from build123d import *

# Parameters (mm, degrees)
F1_DEPTH = 406.4
F2_R     = 1.27
F4_D     = 4.318
F4_DEPTH = 25.4
F4_TIP   = 1.2972580765


with BuildPart() as f1:
    # F0 (on Top) → F1 (new body)
    with BuildSketch(Plane.XY):
        Polygon((12.7, 0), (0, 0), (-12.7, 0), (-12.7, -3.175), (-1.5875, -3.175), (-1.5875, -12.7), (0, -12.7), (1.5875, -12.7), (1.5875, -3.175), (12.7, -3.175), align=None)
    extrude(amount=F1_DEPTH)

    # F2
    f2_edges = [f1.edges().sort_by_distance(p)[0] for p in [
        (-1.5875, -3.175, 203.2),
        (1.5875, -3.175, 203.2),
    ]]
    fillet(f2_edges, radius=F2_R)

    # F4
    with Locations(Plane(origin=(0, 0, 0), x_dir=(-1, 0, 0), z_dir=(0, 1, 0))):
        with Locations((-6.35, 400.05), (-6.35, 387.35), (6.35, 387.35), (6.35, 400.05), (-6.35, 6.35), (-6.35, 19.05), (6.35, 19.05), (6.35, 6.35)):
            Hole(F4_D / 2, depth=F4_DEPTH)
            with Locations((0, 0, -(F4_DEPTH + F4_TIP / 2))):  # 118° drill point
                Cone(0, F4_D / 2, F4_TIP, mode=Mode.SUBTRACT)


solid = f1.part
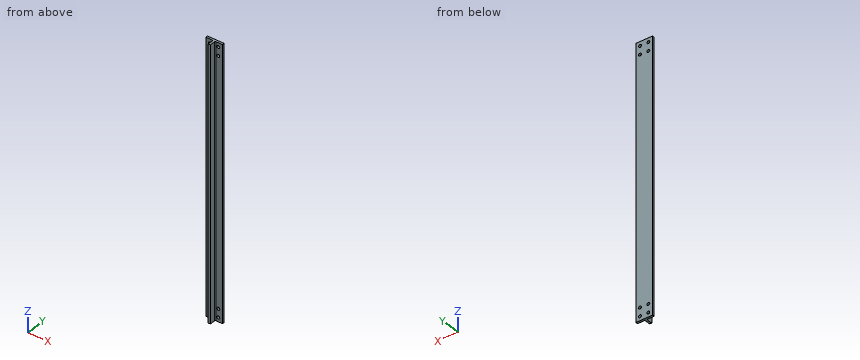
Source: CAD feature listing. Evaluate the final solid. Frame: model axes, mm. Coordinates: 2 decimals unless noted, no trailing zeros. Loops run counter-clockwise (first coordinate to the right, second up) from the corner with the lowest first, then second, coordinate; pieces in that order, holes last. Notation, with made-up numbers: (2, 19) -> (23, 19) arc R27 cw to (23, 45) -> close; hole circle Ø3 at (-14, 36). An arc over 180 degrees is marked (long way). Answer in a Markdown table with one row per item. Add a question column.
Q1. Contact query for flat-ended pins moving along their axis: pin 1 Ø5 at (x, z) = (-7, 261.5) entering from -Y (3 decimals); pin 2 Ø2.5 at (x, z) = (-6.35, 387.35) entering from -Y; pin 3 Ø1 at (y, z) = (-4, 206.5) entering from -X; pin 4 Ø4 at (y, z) = (-7, 286.5) entering from +X. Output: stop coordinate, or through.
Q2. Section B-B on y = -6.75. Return the cut outline in (x, z), and give its area (3 significant figures).
Q3. Ray query, line 1 along X through (y, z) = (-1.8, 400.05); line 2 along Z through (x, y) = (6.35, -2.15); line 3 along Y through (x, z) = (9, 365.5) (3 decimals). Return the intervals inside material, ascending.
Q4. Section A-A on z = 284. Return the cut outline in (x, y) (1 decimal).
Computed values:
| question | item | result |
|---|---|---|
| 1 | pin 1 | stops at y = -3.175 |
| 1 | pin 2 | passes through |
| 1 | pin 3 | stops at x = -2.01 |
| 1 | pin 4 | stops at x = 1.59 |
| 2 | outline | (-1.59, 0) -> (1.59, 0) -> (1.59, 406.4) -> (-1.59, 406.4) -> close |
| 2 | area | 1,290 mm^2 |
| 3 | line 1 | x = -12.7 to -8.51, -4.19 to 4.19, 8.51 to 12.7 |
| 3 | line 2 | z = 0 to 4.19, 8.51 to 16.89, 21.21 to 385.19, 389.51 to 397.89, 402.21 to 406.4 |
| 3 | line 3 | y = -3.175 to 0 |
| 4 | outline | (-12.7, -3.2) -> (-2.9, -3.2) arc R1.3 cw to (-1.6, -4.4) -> (-1.6, -12.7) -> (1.6, -12.7) -> (1.6, -4.4) arc R1.3 cw to (2.9, -3.2) -> (12.7, -3.2) -> (12.7, 0) -> (-12.7, 0) -> close |
